Can you work these out from the model? Positions are in its coordinate system, mm. Face numbers are marked on the shaded views. A direction names the side the tool comes from. Round coordinates to 2 decimals unless told otherwise and drop trailing zeros. Write each loop counter-clockwise with the first axis right and the second up, starting at its lowest first coordinate (ties: lowest second). Pieces come first, ordered by that corner, then holes. Notation, with made-up numbers: M 34,-36 L 72,-36 A13 cw 72,-21 Z; hole C 28,56 d6. An arc over 180 degrees is marked long. Answer in a Markdown table with one row per item. Add a question column.
(1) For the marked faces 1, 2, 3 and 4, which set-ups out of +Z, -Z, +X, -X, +Y, -Y let a thin tool reach every point of the face, with its end or its side?
(2) If I drill on probe 1 along Y at (x, z) = (5.25, 0) (1 decimal); probe 2 along X at (y, z) = (5.75, 3.75) (3 decimals); probe 3 along Z at (x, y) = (1.25, 2.5), over which ranges is the centre line in solid material (lowest first)?
(3) Suppose I cut it at D-D, the plane x = 2.5. Write out the boundary of the cut face in (y, z) (1 decimal).
(4) I'm going to push flat-ended pins straight in: pin 1 (2.5 mm diameter, centred on x = 10.5, y = -6, fed in from +Z); pin 2 (1.8 mm diameter, centred on x = 10, z = 5.5, fed in from +Y); pin 3 (1.3 mm diameter, centred on y = 4.5, z = 0, fed in from +X); pin 4 (5 mm diameter, centred on y = 1.5, z = -1, fed in from +X). Where does each tip first touch, or does it pass through?
(5) Suppose I cut it at C-C, the plane x = 11. Write out the boundary of the cut face in (y, z) (1 decimal).
(6) If we mould it in two halves opening along Y, with no side actions, what happens to the marked faces 5, 6 and 7? For each: released by +Y, released by -Y, zero draft, split by the parting line, or undercut.
(7) Suppose I cut it at A-A, the plane y = 0. Write out the boundary of the cut face in (x, z) (1 decimal), then the cut area to 3 significant figures.
from build123d import *

# Parameters (mm, degrees)
SKETCH2_R          = 4.445
CUT_EXTRUDE1_DEPTH = 18.034
SKETCH5_W          = 8.382
SKETCH5_H          = 2.2225
CUT_EXTRUDE2_DEPTH = 19.496929813
CIRPATTERN1_COUNT  = 4


with BuildPart() as part:
    # Sketch1 → Revolve1 (revolve)
    with BuildSketch(Plane.XY, mode=Mode.PRIVATE) as revolve1_sk:
        with BuildLine():
            Line((0, 0), (13.97, 0))
            Line((13.97, 0), (13.97, 5.715))
            ThreePointArc((13.97, 5.715), (13.109377289, 6.575622711), (12.248754579, 5.715))
            Line((12.248754579, 5.715), (12.248754579, 5.3975))
            Line((12.248754579, 5.3975), (3.175, 5.3975))
            Line((3.175, 5.3975), (3.175, 8.5725))
            Line((3.175, 8.5725), (0, 8.5725))
            Line((0, 8.5725), (0, 0))
        make_face()
    revolve(revolve1_sk.sketch.rotate(Axis((0, 0, 0), (1, 0, 0)), 90), axis=Axis((0, 0, 0), (1, 0, 0)))

    # Sketch2 → Cut-Extrude1 (cut)
    with BuildSketch(Plane.ZY):
        Circle(SKETCH2_R)
    extrude(amount=-CUT_EXTRUDE1_DEPTH, mode=Mode.SUBTRACT)

    # Sketch5 → Cut-Extrude2 (cut, through all)
    with BuildSketch(Plane.XY):
        with Locations((9.779, 0.408848188)):
            Rectangle(SKETCH5_W, SKETCH5_H)
    cut_extrude2 = extrude(amount=-CUT_EXTRUDE2_DEPTH, mode=Mode.SUBTRACT)

    # CirPattern1: Cut-Extrude2 ×4 about axis
    cirpattern1_axis = Axis((0, 0, 0), (1, 0, 0))
    for i in range(1, CIRPATTERN1_COUNT):
        add(cut_extrude2.rotate(cirpattern1_axis, i * 360 / CIRPATTERN1_COUNT), mode=Mode.SUBTRACT)


solid = part.part
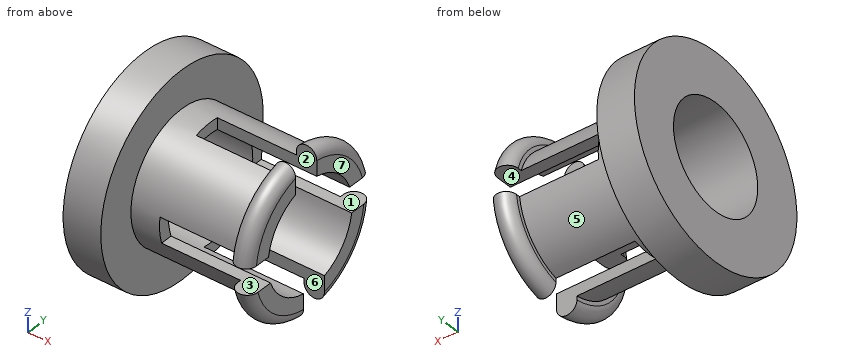
Calculated:
| question | item | result |
|---|---|---|
| 1 | face 1 | +X, +Y, -Y |
| 1 | face 2 | +Z, -Z, +X |
| 1 | face 3 | +X, -Y |
| 1 | face 4 | +X, +Y |
| 2 | probe 1 | -5.4 to -4.4, 4.4 to 5.4 |
| 2 | probe 2 | 0 to 3.175 |
| 2 | probe 3 | -8.2 to -3.68, 3.68 to 8.2 |
| 3 | outline | C 0,0 d17.1; hole C 0,0 d8.9 |
| 4 | pin 1 | z = 2.56 |
| 4 | pin 2 | y = 2.82 |
| 4 | pin 3 | x = 5.59 |
| 4 | pin 4 | through |
| 5 | outline | M -5.4,0.7 L -4.4,0.7 A4.4 cw -1.5,4.2 L -1.5,5.2 A5.4 ccw Z; M -5.2,-1.5 A5.4 ccw -0.7,-5.4 L -0.7,-4.4 A4.4 cw -4.2,-1.5 Z; M 0.7,4.4 A4.4 cw 4.2,1.5 L 5.2,1.5 A5.4 ccw 0.7,5.4 Z; M 1.5,-5.2 A5.4 ccw 5.4,-0.7 L 4.4,-0.7 A4.4 cw 1.5,-4.2 Z |
| 6 | face 5 | split by the parting line |
| 6 | face 6 | undercut |
| 6 | face 7 | zero draft |
| 7 | outline | M 0,-8.6 L 3.2,-8.6 L 3.2,-5.4 L 5.6,-5.4 L 5.6,-4.4 L 0,-4.4 Z; M 0,4.4 L 5.6,4.4 L 5.6,5.4 L 3.2,5.4 L 3.2,8.6 L 0,8.6 Z |
| 7 | area | 30.8 mm² |
